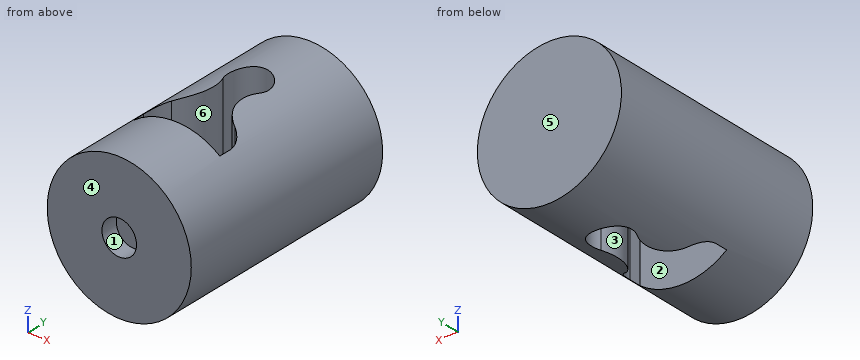
```python
from build123d import *

# Parameters (mm, degrees)
SKETCH2_R               = 12.5
BOSS_EXTRUDE1_DEPTH     = 20
CUT_EXTRUDE1_DEPTH      = 13.5
CUT_EXTRUDE1_DEPTH_BACK = 13.5
SKETCH4_R               = 3
CUT_EXTRUDE2_DEPTH      = 3


with BuildPart() as part:
    # Sketch2 → Boss-Extrude1 (new body, symmetric)
    with BuildSketch(Plane(origin=(0, 0, 0), x_dir=(1, 0, 0), z_dir=(0, 1, 0))):
        Circle(SKETCH2_R)
    extrude(amount=BOSS_EXTRUDE1_DEPTH, both=True)

    # Sketch3 → Cut-Extrude1 (cut, two sides)
    with BuildSketch(Plane.XY) as cut_extrude1_sk:
        with BuildLine():
            Line((-7.5, -8), (7.5, -8))
            Line((7.5, -8), (7.5, -5.902894725))
            ThreePointArc((7.5, -5.902894725), (6.964101615, -3.902894725), (5.5, -2.43879311))
            ThreePointArc((5.5, -2.43879311), (2.754189416, 1.029452854), (3.131578947, 5.436921852))
            ThreePointArc((3.131578947, 5.436921852), (0, 10.5), (-3.131578947, 5.436921852))
            ThreePointArc((-3.131578947, 5.436921852), (-2.754189416, 1.029452854), (-5.5, -2.43879311))
            ThreePointArc((-5.5, -2.43879311), (-6.964101615, -3.902894725), (-7.5, -5.902894725))
            Line((-7.5, -5.902894725), (-7.5, -8))
        make_face()
    extrude(amount=CUT_EXTRUDE1_DEPTH, mode=Mode.SUBTRACT)
    extrude(cut_extrude1_sk.sketch, amount=-CUT_EXTRUDE1_DEPTH_BACK, mode=Mode.SUBTRACT)

    # Sketch4 → Cut-Extrude2 (cut)
    with BuildSketch(Plane(origin=(0, -20, 0), x_dir=(-1, 0, 0), z_dir=(0, -1, 0))):
        Circle(SKETCH4_R)
    extrude(amount=-CUT_EXTRUDE2_DEPTH, mode=Mode.SUBTRACT)


solid = part.part
```
Design review of the part built by this model. Coordinates are the model's own, in mm. Face numbers are marked on the shaded views. A direction names the side the tool comes from. Round coordinates to 2 decimals unless told otherwise and drop trailing zeros. Order: outer loops, then holes, each group sorted by start corner. A loop starts at its lowest first (then second) coordinate and runs counter-clockwise, first axis right, second up. Notation, with made-up numbers: (-6, -37.5) - (32, -37.5) arc R26 cw to (32, -13.5) - close; hole circle Ø2 at (-21.5, 79.5). An arc over 180 degrees is marked (long way). One line per question, with ' | ' between items.
Item 1: Take a section at D-D, the plane z = 10.5. Write out the cut boundary in (x, y), then the cut area to 3 significant figures.
Checks:
outline: (-6.78, -20) - (6.78, -20) - (6.78, -8) - (-6.78, -8) - close; (-6.78, -3.62) arc R4 cw to (-5.5, -2.44) arc R6 ccw to (-3.13, 5.44) arc R3.5 cw (long way) to (3.13, 5.44) arc R6 ccw to (5.5, -2.44) arc R4 cw to (6.78, -3.62) - (6.78, 20) - (-6.78, 20) - close | area: 389 mm²
Item 2: Take a section at A-A, the plane x = 0. Write out the cut boundary in (y, z).
Checks:
outline: (-20, -12.5) - (-8, -12.5) - (-8, 12.5) - (-20, 12.5) - (-20, 3) - (-17, 3) - (-17, -3) - (-20, -3) - close; (10.5, -12.5) - (20, -12.5) - (20, 12.5) - (10.5, 12.5) - close
Item 3: Draft analysis for pull direction Y (two halves, no side actions). For the marked faces 1, 2, 3 and 4, state which applies: +Y half, -Y half, draft (parallel to the pull), parting line (faces both ways), or undercut.
Checks:
face 1: draft | face 2: undercut | face 3: undercut | face 4: -Y half
Item 4: Take a section at C-C, the plane z = -6. Write out the cut boundary in (x, y).
Checks:
outline: (-10.97, -20) - (10.97, -20) - (10.97, 20) - (-10.97, 20) - close; hole (-7.5, -8) - (7.5, -8) - (7.5, -5.9) arc R4 ccw to (5.5, -2.44) arc R6 cw to (3.13, 5.44) arc R3.5 ccw (long way) to (-3.13, 5.44) arc R6 cw to (-5.5, -2.44) arc R4 ccw to (-7.5, -5.9) - close
Item 5: Take a section at B-B, the plane y = 7. Write out the cut boundary in (x, z).
Checks:
outline: (-3.5, -12) - (-3.5, 12) arc R12.5 ccw to start; (3.5, -12) arc R12.5 ccw to (3.5, 12) - close
Item 6: Machinability: for the marked faces 5 and 6, which of the approach directions +Z, -Z, +X, -X, +Y, -Y give a long, thin tool a straight path to every point of the face, cutting with its end or side? Answer none if there is none.
Checks:
face 5: +Z, -Z, +X, -X, +Y | face 6: +Z, -Z
Item 7: Wall thickness on line 1 (X direction, y = -19.35, z = 0); line 2 (Y direction, x = 0, z = 6.75); line 3 (Y direction, x = -5.5, z = -1.25): over which ranges is each line inside the solid? List them lowest first. Write a range as [from, to].
Checks:
line 1: [-12.5, -3], [3, 12.5] | line 2: [-20, -8], [10.5, 20] | line 3: [-20, -8], [-2.44, 20]
Item 8: For P1, Ø1, axis at x = -7, y = -14, coming from the +Z side; P2, Ø2.5, axis at y = -7, z = -1.5, coming from the +X side; P3, Ø10, axis at x = -10, y = 12.5, coming from the -Z side, all flat-tipped, find the tip position at first contact; note any pin that passes through.
Checks:
P1: z = 10.68 | P2: x = 12.5 | P3: z = -11.46
